Verification items for the finished model (mm, model axes). Face numbers are marked on the shaded views. A direction names the side the tool comes from. Round coordinates to 2 decimals unless told otherwise and drop trailing zeros. Write each loop counter-clockwise with the first axis right and the second up, starting at its lowest first coordinate (ties: lowest second). Pieces come first, ordered by that corner, then holes. Notation, with made-up numbers: (28.5, -13) - (76.5, -13) arc R16 cw to (76.5, -4) - close; hole circle Ø8 at (51.25, 31). An arc over 180 degrees is marked (long way). Answer as a JSON object with one key per item and string values. Group by question number.
1) Go/stop test with flat-tipped pins: pin 1 Ø5 at (y, z) = (12.5, 11.5) entering from +X; pin 2 Ø1 at (x, z) = (-26.5, 9.5) entering from -Y; pin 3 Ø8 at (y, z) = (25.5, 8) entering from -X. Record where each tip stops, or that it passes through.
2) Set-up check for the marked faces 4 and 5: record each of +Z, -Z, +X, -X, +Y, -Y from which the full face is reachable in a straight line by a thin tool's end or side.
3) Mould release check, pull along Y, two halves, no side actions. Record for the marked faces 1, 2 and 3: +Y half, -Y half, draft (parallel to the pull), parting line (faces both ways), or undercut.
4) Section check B-B (x = 0). Enter the section's corners in (y, z).
5) Thickness scan on line 1 (Y direction, x = 0, z = 7.6); line 2 (Y direction, x = 0, z = 10.5); line 3 (Y direction, x = 0, z = 4.75). Record the ranges inside material, lowest first.
6) Section check D-D (y = 40). Enter the section's corners in (x, z).
7) Section check C-C (z = 15.25). Enter the section's corners in (x, y).
8) Section check A-A (y = 0). Enter the section's corners in (x, z), then the cut area to 3 significant figures.
Autodesk Inventor part; units mm, degrees
ref_plane "YZ Plane" through (0, 0, 0) normal (1, 0, 0) x (0, 1, 0)
ref_plane "XZ Plane" through (0, 0, 0) normal (0, 1, 0) x (-1, 0, 0)
ref_plane "XY Plane" through (0, 0, 0) normal (0, 0, 1) x (1, 0, 0)
sketch "Эскиз1" plane through (0, 0, 0) normal (0, 0, 1) x (1, 0, 0)
  circle A0 centre (0, 0) radius 55
  circle A1 centre (0, 0) radius 20
  circle A2 centre (0, 40) radius 7
  circle A3 centre (0, -40) radius 7
  dimension "d0" = 110
  dimension "d1" = 40
  dimension "d3" = 14
  dimension "d6" = 360
extrude "Выдавливание1" add sketch "Эскиз1" along normal blind 20
sketch "Эскиз2" plane through (0, 0, 20) normal (0, 0, 1) x (1, 0, 0)
  circle A0 centre (0, 0) radius 55
  circle A1 centre (0, 0) radius 29
  dimension "d10" = 58
extrude "Выдавливание2" cut sketch "Эскиз2" against normal blind 10
chamfer "Фаска1" distance 2.5 angle 45 1 edges at (-29, 0, 20)
chamfer "Фаска2" distance 5.2 angle 45 1 edges at (-7, -40, 0)
chamfer "Фаска3" distance 5.2 angle 45 1 edges at (-7, 40, 0)
properties part number "Крышка"
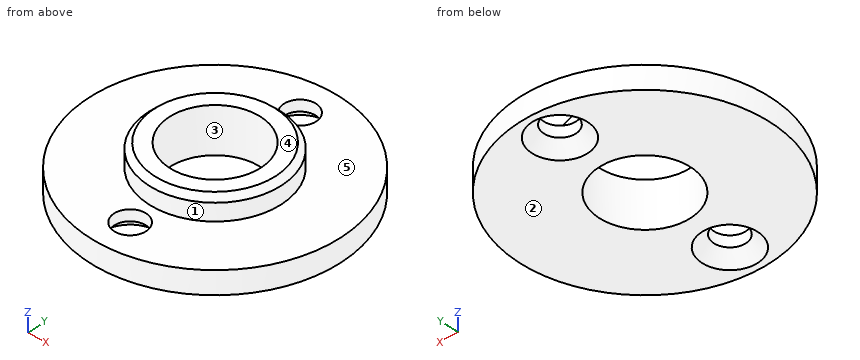
Returned:
{
 "1": {"pin 1": "x = 53.99", "pin 2": "y = -48.47", "pin 3": "x = -50.62"},
 "2": {"face 4": "+Z, +X, -X, +Y, -Y", "face 5": "+Z"},
 "3": {"face 1": "parting line", "face 2": "draft", "face 3": "undercut"},
 "4": {"outline": "(-55, 0) - (-52.2, 0) - (-47, 5.2) - (-47, 10) - (-55, 10) - close; (-33, 5.2) - (-27.8, 0) - (-20, 0) - (-20, 20) - (-26.5, 20) - (-29, 17.5) - (-29, 10) - (-33, 10) - close; (20, 0) - (27.8, 0) - (33, 5.2) - (33, 10) - (29, 10) - (29, 17.5) - (26.5, 20) - (20, 20) - close; (47, 5.2) - (52.2, 0) - (55, 0) - (55, 10) - (47, 10) - close"},
 "5": {"line 1": "-55 to -47, -33 to -20, 20 to 33, 47 to 55", "line 2": "-29 to -20, 20 to 29", "line 3": "-55 to -47.45, -32.55 to -20, 20 to 32.55, 47.45 to 55"},
 "6": {"outline": "(-37.75, 0) - (-12.2, 0) - (-7, 5.2) - (-7, 10) - (-37.75, 10) - close; (7, 5.2) - (12.2, 0) - (37.75, 0) - (37.75, 10) - (7, 10) - close"},
 "7": {"outline": "circle Ø58 at (0, 0); hole circle Ø40 at (0, 0)"},
 "8": {"outline": "(-55, 0) - (-20, 0) - (-20, 20) - (-26.5, 20) - (-29, 17.5) - (-29, 10) - (-55, 10) - close; (20, 0) - (55, 0) - (55, 10) - (29, 10) - (29, 17.5) - (26.5, 20) - (20, 20) - close", "area": "874 mm2"}
}
